Design review of the part built by this model. Coordinates are the model's own, in mm. Face numbers are marked on the shaded views. A direction names the side the tool comes from. Coordinates: 2 decimals unless noted, no trailing zeros. Order: outer loops, then holes, each group sorted by start corner. A loop starts at its lowest first (then second) coordinate and runs counter-clockwise, first axis right, second up. Notation, with made-up numbers: (-26, -3) -> (-7, -3) arc R11 cw to (-7, 13) -> close; hole circle Ø3 at (-2.5, -36). An arc over 180 degrees is marked (long way). Use a Markdown table: item, result. Add a question column.
Q1. Machinability: for the marked faces 1 and 2, which of the approach directions +Z, -Z, +X, -X, +Y, -Y give a long, thin tool a straight path to every point of the face, cutting with its end or side? Answer none if there is none.
Q2. Wall thickness on probe 1 along X at (y, z) = (1, 0); probe 2 along X at (y, z) = (31.5, -15); probe 3 along Y at (x, z) = (8.5, -10): over which ranges is each line inside the solid? List them lowest first.
Q3. Add section A-A (z = 0). State the section outline as (x, y) points.
Q4. Insertion check: pin 1 (21 mm diameter, centred on x = -7, y = 19, fed in from +Z). The pin has a flat end and moves straight along its axis. Give the tip position at first contact, or say it passes through.
Q5. Add section B-B (x = -15). State the section outline as (y, z) points, then the cut area to 3 significant figures.
Q6. Add section C-C (z = 8). State the section outline as (x, y) points.
Q7. The part is to be moulded in two halves that separate along X. For the marked faces 3, 4 and 5, say which applies: pulls with the +X half, pulls with the -X half, needs draft (parallel to the pull), parting line crosses it, or undercut.
Q8. Add section D-D (y = 20). State the section outline as (x, z) points.
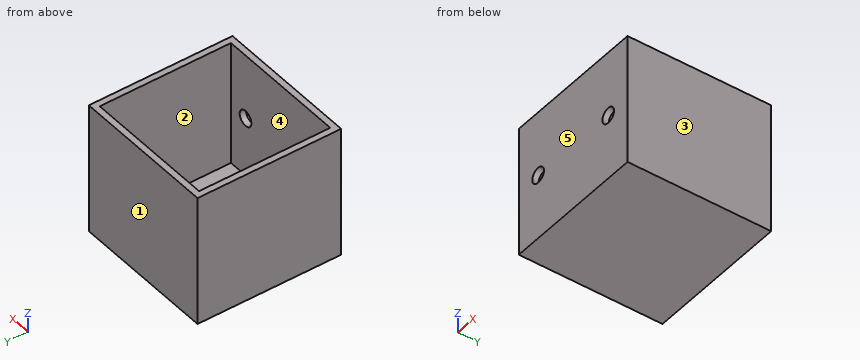
from build123d import *

# Parameters (mm, degrees)
SKETCH2_W           = 46.5
SKETCH2_H           = 42.2
SKETCH2_R           = 2.5
BOSS_EXTRUDE1_DEPTH = 2
BOSS_EXTRUDE2_DEPTH = 42.2
SKETCH4_W           = 46.5
SKETCH4_H           = 42.2
BOSS_EXTRUDE3_DEPTH = 2


with BuildPart() as part:
    # Sketch2 → Boss-Extrude1 (new body)
    with BuildSketch(Plane(origin=(0, 0, 0), x_dir=(1, 0, 0), z_dir=(0, 1, 0))):
        Rectangle(SKETCH2_W, SKETCH2_H)
        with Locations(Location((-15, 0, 0), (0, 0, 270))):
            Circle(SKETCH2_R, mode=Mode.SUBTRACT)
        with Locations(Location((15, 0, 0), (0, 0, 90))):
            Circle(SKETCH2_R, mode=Mode.SUBTRACT)
    extrude(amount=BOSS_EXTRUDE1_DEPTH)

    # Sketch3 → Boss-Extrude2 (add)
    with BuildSketch(Plane(origin=(0, 2, 0), x_dir=(1, 0, 0), z_dir=(0, 1, 0))):
        Polygon((-23.25, -21.1), (-21.25, -21.1), (-21.25, 19.1), (21.25, 19.1), (21.25, -21.1), (23.25, -21.1), (23.25, 21.1), (-23.25, 21.1), align=None)
    extrude(amount=BOSS_EXTRUDE2_DEPTH)

    # Sketch4 → Boss-Extrude3 (add)
    with BuildSketch(Plane(origin=(0, 44.2, 0), x_dir=(1, 0, 0), z_dir=(0, 1, 0))):
        Rectangle(SKETCH4_W, SKETCH4_H)
    extrude(amount=BOSS_EXTRUDE3_DEPTH)


solid = part.part
Established:
| question | item | result |
|---|---|---|
| 1 | face 1 | +Z, -Z, +X, -X, +Y |
| 1 | face 2 | +Z |
| 2 | probe 1 | -23.25 to -17.5, -12.5 to 12.5, 17.5 to 23.25 |
| 2 | probe 2 | -23.25 to -21.25, 21.25 to 23.25 |
| 2 | probe 3 | 0 to 2, 44.2 to 46.2 |
| 3 | outline | (-23.25, 0) -> (-17.5, 0) -> (-17.5, 2) -> (-21.25, 2) -> (-21.25, 44.2) -> (21.25, 44.2) -> (21.25, 2) -> (17.5, 2) -> (17.5, 0) -> (23.25, 0) -> (23.25, 46.2) -> (-23.25, 46.2) -> close; (-12.5, 0) -> (12.5, 0) -> (12.5, 2) -> (-12.5, 2) -> close |
| 4 | pin 1 | z = -19.1 |
| 5 | outline | (0, -21.1) -> (46.2, -21.1) -> (46.2, 21.1) -> (44.2, 21.1) -> (44.2, -19.1) -> (2, -19.1) -> (2, -2.5) -> (0, -2.5) -> close; (0, 2.5) -> (2, 2.5) -> (2, 21.1) -> (0, 21.1) -> close |
| 5 | area | 243 mm^2 |
| 6 | outline | (-23.25, 0) -> (23.25, 0) -> (23.25, 46.2) -> (-23.25, 46.2) -> close; hole (-21.25, 2) -> (21.25, 2) -> (21.25, 44.2) -> (-21.25, 44.2) -> close |
| 7 | face 3 | pulls with the +X half |
| 7 | face 4 | undercut |
| 7 | face 5 | needs draft |
| 8 | outline | (-23.25, -21.1) -> (23.25, -21.1) -> (23.25, 21.1) -> (21.25, 21.1) -> (21.25, -19.1) -> (-21.25, -19.1) -> (-21.25, 21.1) -> (-23.25, 21.1) -> close |
